```python
from build123d import *

# Parameters (mm, degrees)
F0_R       = 725.116012299
F1_DEPTH   = 962.66
F2_R       = 446.733222467
F1_FACE1_R = 725.116012299
F4_R       = 404.6577748379
F5_DEPTH   = 962.66


with BuildPart() as f1:
    # F0 (on Top) → F1 (new body)
    with BuildSketch(Plane.XY):
        Circle(F0_R)
    extrude(amount=F1_DEPTH)

    # F2 (on face) → F3 section 0
    with BuildSketch(Plane.XY.offset(962.66)):
        Circle(F2_R)
    # F1_face1 (on face) → F3 section 1
    with BuildSketch(Plane(origin=(0, 0, 0), x_dir=(1, 0, 0), z_dir=(0, 0, -1))):
        Circle(F1_FACE1_R)
    loft(mode=Mode.INTERSECT)

    # F4
    f4_edges = [f1.edges().sort_by_distance(p)[0] for p in [
        (-446.733222, 0, 962.66),
    ]]
    fillet(f4_edges, radius=F4_R)

    # F5 (cut): a face of the model
    f5_faces = [f1.faces().sort_by_distance(p)[0] for p in [
        (0, 0, 962.66),
    ]]
    extrude(f5_faces, amount=-F5_DEPTH, mode=Mode.SUBTRACT)


solid = f1.part
```
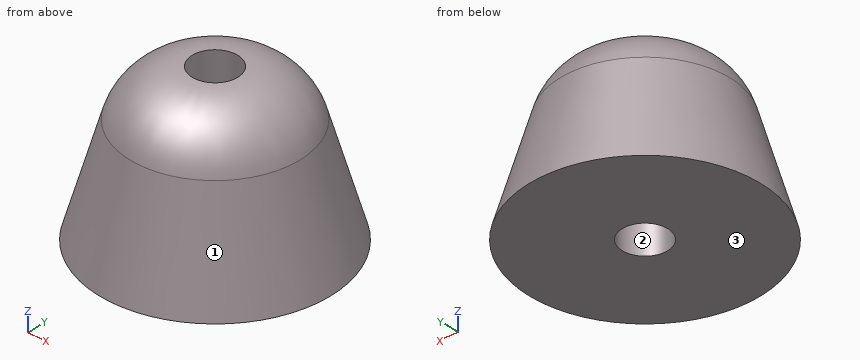
Can you work these out from the model? Positions are in its coordinate system, mm. Face numbers are marked on the shaded views. Coordinates: 2 decimals unless noted, no trailing zeros. Write each loop counter-clockwise with the first axis right and the second up, starting at its lowest first coordinate (ties: lowest second). Pieces come first, ordered by that corner, then holes. Notation, with made-up numbers: M 76,49.25 L 127,49.25 A11 ccw 127,68.25 Z; hole C -36,42.25 d4. An arc over 180 degrees is marked long. Write item = value, one per line. Start each with the question number.
Q1. If I drill on L1, parallel to Y at x = -82, z = 182; L2, parallel to Y at x = 0, z = 473; L3, parallel to X at y = 61, z = 351.5, over which ranges is the centre line in solid material (lowest first)? Write a range as [from, to].
Q2. Thinking about a two-plate mould opening in X: for the marked faces 1, 2 and 3, which applies, released by +X, released by -X, zero draft, split by the parting line, or undercut?
Q3. I'm going to push flat-ended pins straight in: pin 1 (2 mm diameter, centred on x = 349.5, y = -135, fed in from -Z); pin 2 (5 mm diameter, centred on x = -170, z = 606.5, fed in from -Y); pin 3 (5 mm diameter, centred on x = 285, z = 511.5, fed in from +Y); pin 4 (1 mm diameter, centred on y = 438.5, z = 189, fed in from -X). Where does each tip first touch, or does it pass through?
Q4. If we section it at A-A, the plane z = 499: Write out the boundary of the cut face in (x, y).
Check sheet entries:
q1.L1 = [-667.47, -116.56], [116.56, 667.47]
q1.L2 = [-588.33, -142.51], [142.51, 588.33]
q1.L3 = [-620.48, -128.8], [128.8, 620.48]
q2.face_1 = split by the parting line
q2.face_2 = undercut
q2.face_3 = zero draft
q3.pin_1 = 0
q3.pin_2 = -523.89
q3.pin_3 = 503.57
q3.pin_4 = -507.66
q4.outline = C 0,0 d1161.63; hole C 0,0 d285.03
